Geometry: final body of the model. Coordinates: model frame, mm. Face numbers are marked on the shaded views. A direction names the side the tool comes from. Give positions to 0.01 mm unless a question says otherwise; leave off trailing zeros. Order: outer loops, then holes, each group sorted by start corner. A loop starts at its lowest first (then second) coordinate and runs counter-clockwise, first axis right, second up. Notation, with made-up numbers: (2, 31) -> (13, 31) arc R22 cw to (13, 55) -> close; hole circle Ø7 at (76, 47). An arc over 180 degrees is marked (long way). Write item = value, one per line.
```python
from build123d import *

# Parameters (mm, degrees)
ESTRUSIONE_SOTTILE1_DEPTH      = 25
ESTRUSIONE_SOTTILE1_DEPTH_BACK = 25
SCALE2_SCALE                   = 0.93


with BuildPart() as part:
    # Schizzo2 → Estrusione-Sottile1 (new, two sides)
    with BuildSketch(Plane(origin=(-3.626199773, -4.388168382, 0), x_dir=(1, 0, 0), z_dir=(0, 0, 1))) as estrusione_sottile1_sk:
        with BuildLine():
            Line((-226.626080874, -48.830329598), (24.988136504, -38.271646045))
            ThreePointArc((24.988136504, -38.271646045), (61.276185696, -10.897676453), (39.925535167, 29.230947338))
            Line((39.925535167, 29.230947338), (-136.579797, 79.141284263))
            ThreePointArc((-136.579797, 79.141284263), (-161.317329277, 81.14637928), (-184.196927163, 71.52921183))
            Line((-184.196927163, 71.52921183), (-255.562423669, 30.722741893))
            ThreePointArc((-255.562423669, 30.722741893), (-269.023375691, -19.212630891), (-226.626080874, -48.830329598))
        make_face()
        with BuildLine():
            Line((-226.734029631, -43.830459075), (25.044382174, -33.264885303))
            ThreePointArc((25.044382174, -33.264885303), (56.34084272, -10.054333528), (38.316167271, 24.489974706))
            Line((38.316167271, 24.489974706), (-138.050550004, 74.361115557))
            ThreePointArc((-138.050550004, 74.361115557), (-160.616278185, 76.194878875), (-181.452431457, 67.338836133))
            Line((-181.452431457, 67.338836133), (-252.686438473, 26.607551295))
            ThreePointArc((-252.686438473, 26.607551295), (-264.26748414, -17.659406707), (-226.734029631, -43.830459075))
        make_face(mode=Mode.SUBTRACT)
    extrude(amount=ESTRUSIONE_SOTTILE1_DEPTH)
    extrude(estrusione_sottile1_sk.sketch, amount=-ESTRUSIONE_SOTTILE1_DEPTH_BACK)


with BuildPart() as part_1:
    # Scale2: scaled about (-111.699071241, 1.574242956, 0)
    add(part.part.scale(SCALE2_SCALE).moved(Location((-7.818934987, 0.110197007, 0))))


solid = part_1.part
```
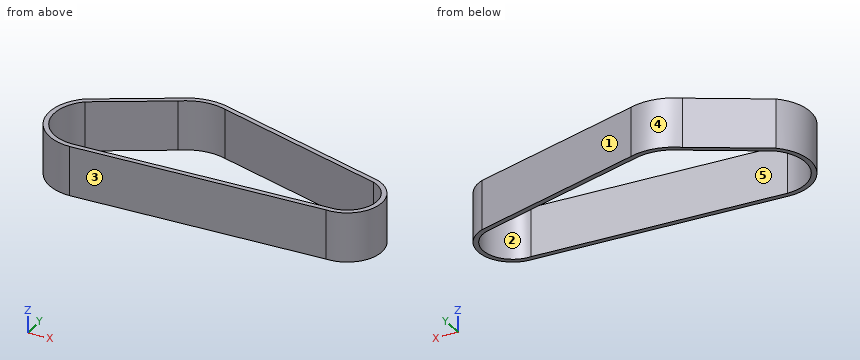
1) Section query C-C (x = -23). Output: boundary loops of the cut face in (y, z), plus the area to 3 significant figures.
Check sheet entries:
outline = (-41.03, -23.25) -> (-36.38, -23.25) -> (-36.38, 23.25) -> (-41.03, 23.25) -> close; (32.22, -23.25) -> (37.05, -23.25) -> (37.05, 23.25) -> (32.22, 23.25) -> close
area = 441 mm²
2) Section query B-B (y = -30.5). Output: boundary loops of the cut face in (x, z).
Check sheet entries:
outline = (-257.04, -23.25) -> (-251.32, -23.25) -> (-251.32, 23.25) -> (-257.04, 23.25) -> close; (29.17, -23.25) -> (36.61, -23.25) -> (36.61, 23.25) -> (29.17, 23.25) -> close
3) Reachability of the marked faces 1 and 2 from +Z, -Z, +X, -X, +Y, -Y: full face, straight path, thin tool, end or side. Return the list, or none.
Check sheet entries:
face_1 = +Z, -Z, +X, +Y
face_2 = +Z, -Z
4) Line query: line 1 (Y direction, x = -41, z = -16); line 2 (Y direction, x = -136, z = 4); line 3 (X direction, y = 1.5, z = -19.5). Output: solid intervals per line, ascending. Write a range as from..to.
Check sheet entries:
line_1 = -41.79..-37.14, 37.31..42.14
line_2 = -45.78..-41.12, 64.17..69.01
line_3 = -262.92..-258.14, 40.56..45.42
5) Section query A-A (z = -9). Output: boundary loops of the cut face in (x, y), plus the area to 3 significant figures.
Check sheet entries:
outline = (-248.86, 24.6) arc R41.85 ccw to (-221.95, -49.38) -> (12.05, -39.56) arc R32.55 ccw to (25.94, 23.21) -> (-138.21, 69.63) arc R48.67 ccw to (-182.49, 62.55) -> close; hole (-246.19, 20.77) arc R37.2 ccw to (-222.05, -44.73) -> (12.1, -34.91) arc R27.9 ccw to (24.44, 18.8) -> (-139.58, 65.19) arc R44.02 ccw to (-179.94, 58.65) -> close
area = 3,290 mm²
6) Mould query, pull axis Y, two halves, no side actions, for the marked faces 3, 4 and 5. Classes: +Y half, -Y half, draft (parallel to the pull), parting line (faces both ways), or undercut.
Check sheet entries:
face_3 = -Y half
face_4 = +Y half
face_5 = undercut
7) First-contact query: P1, Ø3, axis at y = 23.5, z = 9.5, coming from the +X side; P2, Ø6, axis at y = 13, z = -5, coming from the -X side; P3, Ø8, axis at y = 54.5, z = 10, coming from the -X side. Flat tips, straight axial feed; report the tip coordinate or a pass-through.
Check sheet entries:
P1 = 28.65
P2 = -260.05
P3 = -203.57
